from build123d import *

# Parameters (mm, degrees)
BOSS_EXTRUDE1_DEPTH = 20
FILLET1_R           = 5
SKETCH2_R           = 5.5
CUT_EXTRUDE1_DEPTH  = 21
SKETCH3_R           = 9
CUT_EXTRUDE2_DEPTH  = 11


with BuildPart() as part:
    # Sketch1 → Boss-Extrude1 (new body)
    with BuildSketch(Plane(origin=(0, 0, 0), x_dir=(1, 0, 0), z_dir=(0, 1, 0))):
        with BuildLine():
            Line((-115, 70), (-115, -70))
            ThreePointArc((-115, -70), (-109.142135624, -84.142135624), (-95, -90))
            Line((-95, -90), (95, -90))
            ThreePointArc((95, -90), (109.142135624, -84.142135624), (115, -70))
            Line((115, -70), (115, 70))
            ThreePointArc((115, 70), (109.142135624, 84.142135624), (95, 90))
            Line((95, 90), (-95, 90))
            ThreePointArc((-95, 90), (-109.142135624, 84.142135624), (-115, 70))
        make_face()
    extrude(amount=BOSS_EXTRUDE1_DEPTH)

    # Fillet1
    fillet1_edges = [part.edges().sort_by_distance(p)[0] for p in [
        (109.142135624, 20, 84.142135624),
        (115, 20, 0),
        (109.142135624, 20, -84.142135624),
        (0, 20, -90),
        (-109.142135624, 20, -84.142135624),
        (-115, 20, 0),
        (-109.142135624, 20, 84.142135624),
        (0, 20, 90),
    ]]
    fillet(fillet1_edges, radius=FILLET1_R)

    # Sketch2 → Cut-Extrude1 (cut, through all)
    with BuildSketch(Plane(origin=(0, 20, 0), x_dir=(1, 0, 0), z_dir=(0, 1, 0))):
        with Locations((-75, 30)):
            Circle(SKETCH2_R)
        with Locations((75, 30)):
            Circle(SKETCH2_R)
    cut_extrude1 = extrude(amount=-CUT_EXTRUDE1_DEPTH, mode=Mode.SUBTRACT)

    # Sketch3 → Cut-Extrude2 (cut)
    with BuildSketch(Plane.XZ):
        with Locations((-75, -30)):
            Circle(SKETCH3_R)
        with Locations((75, -30)):
            Circle(SKETCH3_R)
    cut_extrude2 = extrude(amount=-CUT_EXTRUDE2_DEPTH, mode=Mode.SUBTRACT)

    # Mirror1: Cut-Extrude1, Cut-Extrude2 across plane
    add(cut_extrude1.mirror(Plane.XY), mode=Mode.SUBTRACT)
    add(cut_extrude2.mirror(Plane.XY), mode=Mode.SUBTRACT)


solid = part.part
Check sheet for the modelled part. Datum: model origin and axes. Units: mm. A direction names the side the tool comes from. Round coordinates to 2 decimals unless told otherwise and drop trailing zeros. Loops run counter-clockwise (first coordinate to the right, second up) from the corner with the lowest first, then second, coordinate; pieces in that order, holes last.
1. Sectioned sample at C-C on y = 3.5. Record the boundary of the cut face in (x, z), and give its area (3 significant figures).
2. Gauge pin test, flat ends, axial feed: pin 1 Ø6.5 at (x, z) = (75, -30) entering from +Y; pin 2 Ø12.5 at (x, z) = (-75, 30) entering from -Y. Record the tip position at first contact, or that the pin passes through.
3. Sectioned sample at A-A on z = 30. Record the boundary of the cut face in (x, y), and give its area (3 significant figures).
4. Scan lines: probe 1 along X at (y, z) = (6, 30); probe 2 along X at (y, z) = (15, -30); probe 3 along Z at (x, y) = (75, 8.5). Record each from-to range of solid material in increasing order.
5. Mould release check, pull along Z, two halves, no side actions. Record for faces 3 (the flat face through (-2, 0, -1)), 4 (the cylindrical face through (-66.416, 5.423, -27.297)), 5 (the cylindrical face through (-109.297, 7.395, 83.986)), 6 (the flat face through (71, 11, 34)): released by +Z, released by -Z, zero draft, split by the parting line, or undercut.
6. Sectioned sample at B-B on x = 75. Record the boundary of the cut face in (y, z).
7. Set-up check for faces 1 (the cylindrical face through (83.584, 5.423, -27.297)), 2 (the cylindrical face through (69.505, 15.563, -30.242)): record each of +Z, -Z, +X, -X, +Y, -Y from which the full face is reachable in a straight line by a thin tool's end or side.
Recorded:
1. outline: (-115, -70) arc R20 ccw to (-95, -90) - (95, -90) arc R20 ccw to (115, -70) - (115, 70) arc R20 ccw to (95, 90) - (-95, 90) arc R20 ccw to (-115, 70) - close; hole circle Ø18 at (-75, -30); hole circle Ø18 at (-75, 30); hole circle Ø18 at (75, -30); hole circle Ø18 at (75, 30)
1. area: 40,000 mm2
2. pin 1: passes through
2. pin 2: stops at y = 11
3. outline: (-115, 0) - (-84, 0) - (-84, 11) - (-80.5, 11) - (-80.5, 20) - (-110, 20) arc R5 ccw to (-115, 15) - close; (-69.5, 11) - (-66, 11) - (-66, 0) - (66, 0) - (66, 11) - (69.5, 11) - (69.5, 20) - (-69.5, 20) - close; (80.5, 11) - (84, 11) - (84, 0) - (115, 0) - (115, 15) arc R5 ccw to (110, 20) - (80.5, 20) - close
3. area: 4,000 mm2
4. probe 1: x = -115 to -84, -66 to 66, 84 to 115
4. probe 2: x = -115 to -80.5, -69.5 to 69.5, 80.5 to 115
4. probe 3: z = -90 to -39, -21 to 21, 39 to 90
5. face 3: zero draft
5. face 4: undercut
5. face 5: released by +Z
5. face 6: undercut
6. outline: (0, -90) - (15, -90) arc R5 ccw to (20, -85) - (20, -35.5) - (11, -35.5) - (11, -39) - (0, -39) - close; (0, -21) - (11, -21) - (11, -24.5) - (20, -24.5) - (20, 24.5) - (11, 24.5) - (11, 21) - (0, 21) - close; (0, 39) - (11, 39) - (11, 35.5) - (20, 35.5) - (20, 85) arc R5 ccw to (15, 90) - (0, 90) - close
7. face 1: -Y
7. face 2: +Y, -Y
